Geometry check sheet. Reference: the model listing, model coordinates, mm. Coordinates: 2 decimals unless noted, no trailing zeros. Loops run counter-clockwise (first coordinate to the right, second up) from the corner with the lowest first, then second, coordinate; pieces in that order, holes last.
from build123d import *

# Parameters (mm, degrees)
F0_W     = 360.6640398502
F0_H     = 159.1658816382
F1_DEPTH = 9.525
F3_D     = 63.5
F4_W     = 159.013863685
F4_H     = 78.3692672849
F5_DEPTH = 9.525


with BuildPart() as f1:
    # F0 (on Top) → F1 (new body)
    with BuildSketch(Plane.XY):
        Rectangle(F0_W, F0_H)
    extrude(amount=F1_DEPTH)

    # F3 (through all)
    with Locations(Plane.XY.offset(9.525)):
        with Locations((0, 0)):
            Hole(F3_D / 2)

    # F4 (on face) → F5 (join)
    with BuildSketch(Plane.YZ.offset(180.3320199251)):
        with Locations((-0.0760089766, -39.1846336424)):
            Rectangle(F4_W, F4_H)
    extrude(amount=-F5_DEPTH)


solid = f1.part
1) Section check C-C on y = -55. Record the cut outline in (x, z) (3 decimals), and give its area (3 significant figures).
Data:
outline: (-180.332, 0) - (170.807, 0) - (170.807, -78.369) - (180.332, -78.369) - (180.332, 9.525) - (-180.332, 9.525) - close
area: 4,180 mm2
2) Section check A-A on x = 0. Record the cut outline in (y, z) (3 decimals).
Data:
outline: (-79.583, 0) - (-31.75, 0) - (-31.75, 9.525) - (-79.583, 9.525) - close; (31.75, 0) - (79.583, 0) - (79.583, 9.525) - (31.75, 9.525) - close
3) Mould release check, pull along X, two halves, no side actions. Record for faces 1 (the cylindrical face through (6.883, -30.995, 4.696)), 2 (the flat face through (170.807, -1, -39)), 3 (the flat face through (180.332, -1, -34)), 4 (the flat face through (-3, 36, 0)): +X half, -X half, draft (parallel to the pull), parting line (faces both ways), or undercut.
Data:
face 1: undercut
face 2: -X half
face 3: +X half
face 4: draft
4) Material ranges on probe 1 along Y at (x, z) = (0, 2.75); probe 2 along X at (y, z) = (15, -73); probe 3 along Z at (x, y) = (-65, 65.5) (3 decimals), recorded low to high.
Data:
probe 1: y = -79.58 to -31.75, 31.75 to 79.58
probe 2: x = 170.81 to 180.33
probe 3: z = 0 to 9.525
5) Section check D-D on z = -8. Record the cut outline in (x, y).
Data:
outline: (170.81, -79.58) - (180.33, -79.58) - (180.33, 79.43) - (170.81, 79.43) - close
6) Section check B-B on y = 0. Record the cut outline in (x, z) (3 decimals).
Data:
outline: (-180.332, 0) - (-31.75, 0) - (-31.75, 9.525) - (-180.332, 9.525) - close; (31.75, 0) - (170.807, 0) - (170.807, -78.369) - (180.332, -78.369) - (180.332, 9.525) - (31.75, 9.525) - close
7) Depth check by flat-ended pin: pin 1 (5 mm diameter, centred on x = -46.5, y = 19, fed in from -Z); pin 2 (10.5 mm diameter, centred on x = 174.5, z = -56.5, fed in from +Y). Enter the tip coordinate at first touch or a pass-through.
Data:
pin 1: stops at z = 0
pin 2: stops at y = 79.43
